Input: part model. Units: mm. Frame: model coordinates. Round coordinates to 2 decimals unless told otherwise and drop trailing zeros. Write each loop counter-clockwise with the first axis right and the second up, starting at its lowest first coordinate (ties: lowest second). Pieces come first, ordered by that corner, then holes. Notation, with made-up numbers: (36.25, -9.5) -> (88.25, -9.5) arc R34 ccw to (88.25, 20.5) -> close; hole circle Ø4 at (-1, 56). An arc over 180 degrees is marked (long way). Write item = value, one per line.
```python
from build123d import *

# Parameters (mm, degrees)
SKETCH1_W               = 249.6
SKETCH1_H               = 340.9
SKETCH1_R               = 2.1
SKETCH1_R_2             = 2.5
SKETCH1_R_3             = 1.59
SKETCH1_R_4             = 12.5
SKETCH1_W_2             = 33
SKETCH1_H_2             = 90
BOSS_EXTRUDE1_DEPTH     = 5
CUT_EXTRUDE3_DEPTH      = 193
CUT_EXTRUDE3_DEPTH_BACK = 193
CUT_EXTRUDE6_DEPTH      = 6
SKETCH8_R               = 2
SKETCH8_R_2             = 2.1
SKETCH8_R_3             = 2.058578644
SKETCH8_R_4             = 4
SKETCH8_R_5             = 4.3
CUT_EXTRUDE7_DEPTH      = 6
SKETCH9_R               = 12.5
SKETCH9_R_2             = 2.1
CUT_EXTRUDE8_DEPTH      = 6


with BuildPart() as part:
    # Sketch1 → Boss-Extrude1 (new body)
    with BuildSketch(Plane.XY):
        with Locations((124.8, -170.45)):
            Rectangle(SKETCH1_W, SKETCH1_H)
        with Locations((104.3, -14)):
            Circle(SKETCH1_R, mode=Mode.SUBTRACT)
        with Locations((245.6, -26.5)):
            Circle(SKETCH1_R_2, mode=Mode.SUBTRACT)
        with Locations((245.6, -77.5)):
            Circle(SKETCH1_R_2, mode=Mode.SUBTRACT)
        with Locations((145.3, -14)):
            Circle(SKETCH1_R, mode=Mode.SUBTRACT)
        with Locations((179.16, -36.375)):
            Circle(SKETCH1_R_3, mode=Mode.SUBTRACT)
        with Locations((179.16, -67.625)):
            Circle(SKETCH1_R_3, mode=Mode.SUBTRACT)
        with Locations((124.8, -14)):
            Circle(SKETCH1_R_4, mode=Mode.SUBTRACT)
        with Locations((141.06, -36.375)):
            Circle(SKETCH1_R_3, mode=Mode.SUBTRACT)
        with Locations((153.76, -36.375)):
            Circle(SKETCH1_R_3, mode=Mode.SUBTRACT)
        with Locations((166.46, -36.375)):
            Circle(SKETCH1_R_3, mode=Mode.SUBTRACT)
        with Locations((141.06, -67.625)):
            Circle(SKETCH1_R_3, mode=Mode.SUBTRACT)
        with Locations((153.76, -67.625)):
            Circle(SKETCH1_R_3, mode=Mode.SUBTRACT)
        with Locations((166.46, -67.625)):
            Circle(SKETCH1_R_3, mode=Mode.SUBTRACT)
        with Locations((83.14, -67.625)):
            Circle(SKETCH1_R_3, mode=Mode.SUBTRACT)
        with Locations((95.84, -67.625)):
            Circle(SKETCH1_R_3, mode=Mode.SUBTRACT)
        with Locations((108.54, -67.625)):
            Circle(SKETCH1_R_3, mode=Mode.SUBTRACT)
        with Locations((83.14, -36.375)):
            Circle(SKETCH1_R_3, mode=Mode.SUBTRACT)
        with Locations((95.84, -36.375)):
            Circle(SKETCH1_R_3, mode=Mode.SUBTRACT)
        with Locations((108.54, -36.375)):
            Circle(SKETCH1_R_3, mode=Mode.SUBTRACT)
        with Locations((70.44, -67.625)):
            Circle(SKETCH1_R_3, mode=Mode.SUBTRACT)
        with Locations((70.44, -36.375)):
            Circle(SKETCH1_R_3, mode=Mode.SUBTRACT)
        with Locations((4, -77.5)):
            Circle(SKETCH1_R_2, mode=Mode.SUBTRACT)
        with Locations((4, -26.5)):
            Circle(SKETCH1_R_2, mode=Mode.SUBTRACT)
        with Locations((201.66, -52)):
            Rectangle(SKETCH1_W_2, SKETCH1_H_2, mode=Mode.SUBTRACT)
        with BuildLine():
            Line((145.8225, -36.375), (145.8225, -41.375))
            ThreePointArc((145.8225, -41.375), (147.41, -42.9625), (148.9975, -41.375))
            Line((148.9975, -41.375), (148.9975, -36.375))
            ThreePointArc((148.9975, -36.375), (147.41, -34.7875), (145.8225, -36.375))
        make_face(mode=Mode.SUBTRACT)
        with BuildLine():
            Line((158.52, -36.375), (158.52, -41.375))
            ThreePointArc((158.52, -41.375), (160.11, -42.965), (161.7, -41.375))
            Line((161.7, -41.375), (161.7, -36.375))
            ThreePointArc((161.7, -36.375), (160.11, -34.785), (158.52, -36.375))
        make_face(mode=Mode.SUBTRACT)
        with BuildLine():
            Line((171.22, -36.375), (171.22, -41.375))
            ThreePointArc((171.22, -41.375), (172.81, -42.965), (174.4, -41.375))
            Line((174.4, -41.375), (174.4, -36.375))
            ThreePointArc((174.4, -36.375), (172.81, -34.785), (171.22, -36.375))
        make_face(mode=Mode.SUBTRACT)
        with BuildLine():
            Line((145.8225, -67.625), (145.8225, -72.625))
            ThreePointArc((145.8225, -72.625), (147.41, -74.2125), (148.9975, -72.625))
            Line((148.9975, -72.625), (148.9975, -67.625))
            ThreePointArc((148.9975, -67.625), (147.41, -66.0375), (145.8225, -67.625))
        make_face(mode=Mode.SUBTRACT)
        with BuildLine():
            Line((158.52, -67.625), (158.52, -72.625))
            ThreePointArc((158.52, -72.625), (160.11, -74.215), (161.7, -72.625))
            Line((161.7, -72.625), (161.7, -67.625))
            ThreePointArc((161.7, -67.625), (160.11, -66.035), (158.52, -67.625))
        make_face(mode=Mode.SUBTRACT)
        with BuildLine():
            Line((171.22, -67.625), (171.22, -72.625))
            ThreePointArc((171.22, -72.625), (172.81, -74.215), (174.4, -72.625))
            Line((174.4, -72.625), (174.4, -67.625))
            ThreePointArc((174.4, -67.625), (172.81, -66.035), (171.22, -67.625))
        make_face(mode=Mode.SUBTRACT)
        with BuildLine():
            Line((103.7775, -36.375), (103.7775, -41.375))
            ThreePointArc((103.7775, -41.375), (102.19, -42.9625), (100.6025, -41.375))
            Line((100.6025, -41.375), (100.6025, -36.375))
            ThreePointArc((100.6025, -36.375), (102.19, -34.7875), (103.7775, -36.375))
        make_face(mode=Mode.SUBTRACT)
        with BuildLine():
            Line((91.08, -36.375), (91.08, -41.375))
            ThreePointArc((91.08, -41.375), (89.49, -42.965), (87.9, -41.375))
            Line((87.9, -41.375), (87.9, -36.375))
            ThreePointArc((87.9, -36.375), (89.49, -34.785), (91.08, -36.375))
        make_face(mode=Mode.SUBTRACT)
        with BuildLine():
            Line((78.38, -36.375), (78.38, -41.375))
            ThreePointArc((78.38, -41.375), (76.79, -42.965), (75.2, -41.375))
            Line((75.2, -41.375), (75.2, -36.375))
            ThreePointArc((75.2, -36.375), (76.79, -34.785), (78.38, -36.375))
        make_face(mode=Mode.SUBTRACT)
        with BuildLine():
            Line((103.7775, -67.625), (103.7775, -72.625))
            ThreePointArc((103.7775, -72.625), (102.19, -74.2125), (100.6025, -72.625))
            Line((100.6025, -72.625), (100.6025, -67.625))
            ThreePointArc((100.6025, -67.625), (102.19, -66.0375), (103.7775, -67.625))
        make_face(mode=Mode.SUBTRACT)
        with BuildLine():
            Line((91.08, -67.625), (91.08, -72.625))
            ThreePointArc((91.08, -72.625), (89.49, -74.215), (87.9, -72.625))
            Line((87.9, -72.625), (87.9, -67.625))
            ThreePointArc((87.9, -67.625), (89.49, -66.035), (91.08, -67.625))
        make_face(mode=Mode.SUBTRACT)
        with BuildLine():
            Line((78.38, -67.625), (78.38, -72.625))
            ThreePointArc((78.38, -72.625), (76.79, -74.215), (75.2, -72.625))
            Line((75.2, -72.625), (75.2, -67.625))
            ThreePointArc((75.2, -67.625), (76.79, -66.035), (78.38, -67.625))
        make_face(mode=Mode.SUBTRACT)
        with Locations((47.94, -52)):
            Rectangle(SKETCH1_W_2, SKETCH1_H_2, mode=Mode.SUBTRACT)
    extrude(amount=BOSS_EXTRUDE1_DEPTH)

    # Sketch4 → Cut-Extrude3 (cut, two sides)
    with BuildSketch(Plane.XY.offset(5)) as cut_extrude3_sk:
        with BuildLine():
            Line((249.6, -161.594545719), (249.6, -280.754609783))
            ThreePointArc((249.6, -280.754609783), (205.980407386, -221.174577751), (249.6, -161.594545719))
        make_face()
    extrude(amount=CUT_EXTRUDE3_DEPTH, mode=Mode.SUBTRACT)
    extrude(cut_extrude3_sk.sketch, amount=-CUT_EXTRUDE3_DEPTH_BACK, mode=Mode.SUBTRACT)

    # Sketch7 → Cut-Extrude6 (cut, through all)
    with BuildSketch(Plane.XY.offset(5)):
        Polygon((249.6, -283.901637295), (232.162192493, -278.37574383), (226.608591706, -274.129323659), (0, -274.129323659), (0, -340.9), (249.6, -340.9), align=None)
    extrude(amount=-CUT_EXTRUDE6_DEPTH, mode=Mode.SUBTRACT)

    # Sketch8 → Cut-Extrude7 (cut, through all)
    with BuildSketch(Plane.XY.offset(5)):
        with Locations((3.765, -141.718358436)):
            Circle(SKETCH8_R)
        with Locations((18.683520247, -121.657507167)):
            Circle(SKETCH8_R_2)
        with Locations((23.825851269, -156.636878683)):
            Circle(SKETCH8_R_2)
        with Locations((37.868447157, -167.079842856)):
            Circle(SKETCH8_R_3)
        with Locations((41.315537027, -154.065713172)):
            Circle(SKETCH8_R_4)
        with Locations((38.744371516, -136.576027414)):
            Circle(SKETCH8_R)
        with Locations((21.254685758, -139.147192925)):
            Circle(SKETCH8_R_5)
        with Locations((52.786967404, -147.018991586)):
            Circle(SKETCH8_R_3)
    extrude(amount=-CUT_EXTRUDE7_DEPTH, mode=Mode.SUBTRACT)

    # Sketch9 → Cut-Extrude8 (cut, through all)
    with BuildSketch(Plane.XY.offset(5)):
        with Locations((62.4, -249.129323659)):
            Circle(SKETCH9_R)
        with Locations((82.9, -249.129323659)):
            Circle(SKETCH9_R_2)
        with Locations((41.9, -249.129323659)):
            Circle(SKETCH9_R_2)
        with Locations((207.7, -249.129323659)):
            Circle(SKETCH9_R_2)
        with Locations((166.7, -249.129323659)):
            Circle(SKETCH9_R_2)
        with Locations((187.2, -249.129323659)):
            Circle(SKETCH9_R)
    extrude(amount=-CUT_EXTRUDE8_DEPTH, mode=Mode.SUBTRACT)


solid = part.part
```
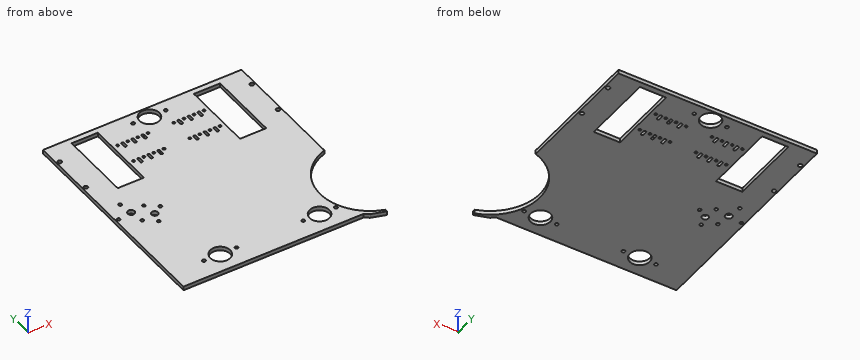
1) Cut plane B-B (x = 122). Return the cut outline in (y, z), and give its area (3 significant figures).
Solutions:
outline = (-274.13, 0) -> (-26.18, 0) -> (-26.18, 5) -> (-274.13, 5) -> close; (-1.82, 0) -> (0, 0) -> (0, 5) -> (-1.82, 5) -> close
area = 1,250 mm^2
2) Cut plane A-A (y = -92). Return the cut outline in (x, z), and give its area (3 significant figures).
Solutions:
outline = (0, 0) -> (31.44, 0) -> (31.44, 5) -> (0, 5) -> close; (64.44, 0) -> (185.16, 0) -> (185.16, 5) -> (64.44, 5) -> close; (218.16, 0) -> (249.6, 0) -> (249.6, 5) -> (218.16, 5) -> close
area = 918 mm^2
3) First-contact query: P1, Ø1.5, axis at x = 180.5, z = 1, coming from the -Y side. Flat tip, straight axial feed; report the tip coordinate or a pass-through.
Solutions:
P1 = -274.13
4) Cut plane C-C (z = 2.75). Count the separate pieces of the cut face and the enclosed holes in it, and give its area (3 significant figures).
Solutions:
separate_pieces = 1
enclosed_holes = 51
area = 56,600 mm^2
5) Line query: L1, parallel to X at y = -32.5, z = 1.85; L2, parallel to Y at x = 95.84, z = 1.85 (3 decimals); L3, parallel to Y at x = 161, z = 0.2. Output: solid intervals per line, ascending. Write a range as from..to.
Solutions:
L1 = 0..31.44, 64.44..185.16, 218.16..249.6
L2 = -274.129..-69.215, -66.035..-37.965, -34.785..0
L3 = -274.13..-73.94, -66.31..-42.69, -35.06..0
6) Cut plane D-D (y = -174). Return the cut outline in (x, z), and give its area (3 significant figures).
Solutions:
outline = (0, 0) -> (227.48, 0) -> (227.48, 5) -> (0, 5) -> close
area = 1,140 mm^2
